```python
from build123d import *

# Parameters (mm, degrees)
BOSS_EXTRUDE1_DEPTH = 25
SKETCH2_R           = 50
BOSS_EXTRUDE2_DEPTH = 25
SKETCH3_R           = 50
CUT_EXTRUDE2_DEPTH  = 25


with BuildPart() as part:
    # Sketch1 → Boss-Extrude1 (new body)
    with BuildSketch(Plane.XY):
        with BuildLine():
            ThreePointArc((-1250, 100), (-1350, 0), (-1250, -100))
            ThreePointArc((-1250, -100), (0, -60.899278339), (1250, -100))
            ThreePointArc((1250, -100), (1350, 0), (1250, 100))
            ThreePointArc((1250, 100), (0, 60.899278339), (-1250, 100))
        make_face()
    extrude(amount=BOSS_EXTRUDE1_DEPTH)

    # Sketch2 → Boss-Extrude2 (add)
    with BuildSketch(Plane(origin=(0, 0, 0), x_dir=(1, 0, 0), z_dir=(0, 0, -1))):
        with Locations((-1250, 0)):
            Circle(SKETCH2_R)
    extrude(amount=BOSS_EXTRUDE2_DEPTH)

    # Sketch3 → Cut-Extrude2 (cut)
    with BuildSketch(Plane.XY.offset(25)):
        with Locations((1250, 0)):
            Circle(SKETCH3_R)
    extrude(amount=-CUT_EXTRUDE2_DEPTH, mode=Mode.SUBTRACT)


solid = part.part
```
Could you check a few things on this model? Use its own coordinates, in mm. Round coordinates to 2 decimals unless told otherwise and drop trailing zeros. Loops run counter-clockwise (first coordinate to the right, second up) from the corner with the lowest first, then second, coordinate; pieces in that order, holes last. Notation, with made-up numbers: (-39.75, 21) -> (11.25, 21) arc R9 cw to (11.25, 38) -> close; hole circle Ø1 at (-14, 51). An arc over 180 degrees is marked (long way). Put each result on its own line as item: value.
Q1. For pin 1 Ø12 at (x, y) = (499, -42) entering from -Z, with a flat end and sliding along its axis, tell me the tip position at first contact or that it passes through.
Checks:
pin 1: z = 0
Q2. I want a section at D-D on x = 198. Write out the boundary of the cut face in (y, z), and give its area (3 significant figures).
Checks:
outline: (-61.88, 0) -> (61.88, 0) -> (61.88, 25) -> (-61.88, 25) -> close
area: 3,090 mm2
Q3. Please list where these lines run through material, in increasing order: line 1 (X direction, y = -4, z = 20); line 2 (Y direction, x = 33, z = 22); line 3 (Z direction, x = -933, y = -25). Write a range as from..to.
Checks:
line 1: -1349.92..1200.16, 1299.84..1349.92
line 2: -60.93..60.93
line 3: 0..25
Q4. I want a section at A-A on y = 0. Write out the boundary of the cut face in (x, z), and give its area (3 significant figures).
Checks:
outline: (-1350, 0) -> (-1300, 0) -> (-1300, -25) -> (-1200, -25) -> (-1200, 0) -> (1200, 0) -> (1200, 25) -> (-1350, 25) -> close; (1300, 0) -> (1350, 0) -> (1350, 25) -> (1300, 25) -> close
area: 67,500 mm2
Q5. I want a section at C-C on x = -951. Write out the boundary of the cut face in (y, z).
Checks:
outline: (-83.52, 0) -> (83.52, 0) -> (83.52, 25) -> (-83.52, 25) -> close
Q6. I want a section at B-B on z = 13. Write out the boundary of the cut face in (x, y), and give its area (3 significant figures).
Checks:
outline: (-1250, -100) arc R20000 cw to (1250, -100) arc R100 ccw to (1250, 100) arc R20000 cw to (-1250, 100) arc R100 ccw to start; hole circle Ø100 at (1250, 0)
area: 393,000 mm2
Q7. Thinking about a two-plate mould opening in X: for faces 1 (the flat face through (-19, 1, 25)), 2 (the cylindrical face through (1297.69, 15.02, 12.68)), 3 (the cylindrical face through (-1202.31, -15.02, -12.32)), 4 (the cylindrical face through (1349.976, -2.199, 12.325)), which applies, pulls with the +X half, pulls with the -X half, needs draft (parallel to the pull), parting line crosses it, or undercut?
Checks:
face 1: needs draft
face 2: undercut
face 3: parting line crosses it
face 4: pulls with the +X half
